from build123d import *

# Parameters (mm, degrees)
BOX001_W          = 40
BOX001_H          = 15
BOX001_DEPTH      = 5
CYLINDER003_R     = 3
CYLINDER003_DEPTH = 6
CYLINDER002_R     = 3
CYLINDER002_DEPTH = 6
CYLINDER001_R     = 1.7
CYLINDER001_DEPTH = 10
CYLINDER_R        = 1.7
CYLINDER_DEPTH    = 10
BOX_W             = 70
BOX_H             = 15
BOX_DEPTH         = 10
FILLET_R          = 2
FILLET001_R       = 2
FILLET002_R       = 7.45


with BuildPart() as cube001:
    # Box001 → Box001 (new body)
    with BuildSketch(Plane(origin=(15, 0, 5), x_dir=(1, 0, 0), z_dir=(0, 0, 1))):
        with Locations((20, 7.5)):
            Rectangle(BOX001_W, BOX001_H)
    extrude(amount=BOX001_DEPTH)


with BuildPart() as sphere001:
    # Sphere001 → Sphere001 (revolve)
    with BuildSketch(Plane(origin=(62.5, 7.5, -2), x_dir=(1, 0, 0), z_dir=(0, -1, 0))):
        with BuildLine():
            ThreePointArc((0, -5), (5, 0), (0, 5))
            Line((0, 5), (0, -5))
        make_face()
    revolve(axis=Axis((62.5, 7.5, -2), (0, 0, 1)))


with BuildPart() as sphere:
    # Sphere → Sphere (revolve)
    with BuildSketch(Plane(origin=(7.5, 7.5, -2), x_dir=(1, 0, 0), z_dir=(0, -1, 0))):
        with BuildLine():
            ThreePointArc((0, -5), (5, 0), (0, 5))
            Line((0, 5), (0, -5))
        make_face()
    revolve(axis=Axis((7.5, 7.5, -2), (0, 0, 1)))


with BuildPart() as cylinder003:
    # Cylinder003 → Cylinder003 (new body)
    with BuildSketch(Plane(origin=(62.5, 7.5, 0), x_dir=(1, 0, 0), z_dir=(0, 0, 1))):
        Circle(CYLINDER003_R)
    extrude(amount=CYLINDER003_DEPTH)


with BuildPart() as cylinder002:
    # Cylinder002 → Cylinder002 (new body)
    with BuildSketch(Plane(origin=(7.5, 7.5, 0), x_dir=(1, 0, 0), z_dir=(0, 0, 1))):
        Circle(CYLINDER002_R)
    extrude(amount=CYLINDER002_DEPTH)


with BuildPart() as cylinder001:
    # Cylinder001 → Cylinder001 (new body)
    with BuildSketch(Plane(origin=(62.5, 7.5, 0), x_dir=(1, 0, 0), z_dir=(0, 0, 1))):
        Circle(CYLINDER001_R)
    extrude(amount=CYLINDER001_DEPTH)


with BuildPart() as cylinder:
    # Cylinder → Cylinder (new body)
    with BuildSketch(Plane(origin=(7.5, 7.5, 0), x_dir=(1, 0, 0), z_dir=(0, 0, 1))):
        Circle(CYLINDER_R)
    extrude(amount=CYLINDER_DEPTH)


with BuildPart() as obj1:
    # Box → Box (new body)
    with BuildSketch(Plane.XY):
        with Locations((35, 7.5)):
            Rectangle(BOX_W, BOX_H)
    extrude(amount=BOX_DEPTH)

    # Fillet
    fillet_edges = [obj1.edges().sort_by_distance(p)[0] for p in [
        (0, 0, 5),
        (0, 15, 5),
        (70, 0, 5),
        (70, 15, 5),
    ]]
    fillet(fillet_edges, radius=FILLET_R)

    # Fillet001
    fillet001_edges = [obj1.edges().sort_by_distance(p)[0] for p in [
        (0, 7.5, 0),
        (0.585786, 0.585786, 0),
        (0.585786, 14.414214, 0),
        (35, 0, 0),
        (35, 15, 0),
        (69.414214, 0.585786, 0),
        (69.414214, 14.414214, 0),
        (70, 7.5, 0),
    ]]
    fillet(fillet001_edges, radius=FILLET001_R)

    # Cut: cut Cylinder
    add(cylinder.part, mode=Mode.SUBTRACT)

    # Cut001: cut Cylinder001
    add(cylinder001.part, mode=Mode.SUBTRACT)

    # Cut002: cut Cylinder002
    add(cylinder002.part, mode=Mode.SUBTRACT)

    # Cut003: cut Cylinder003
    add(cylinder003.part, mode=Mode.SUBTRACT)

    # Cut004: cut Sphere
    add(sphere.part, mode=Mode.SUBTRACT)

    # Cut005: cut Sphere001
    add(sphere001.part, mode=Mode.SUBTRACT)

    # Cut006: cut Cube001
    add(cube001.part, mode=Mode.SUBTRACT)

    # Fillet002
    fillet002_edges = [obj1.edges().sort_by_distance(p)[0] for p in [
        (55, 0, 7.5),
        (15, 0, 7.5),
        (55, 15, 7.5),
        (15, 15, 7.5),
    ]]
    fillet(fillet002_edges, radius=FILLET002_R)


solid = obj1.part
Could you check a few things on this model? Use its own coordinates, in mm. A direction names the side the tool comes from. Round coordinates to 2 decimals unless told otherwise and drop trailing zeros. Write each loop counter-clockwise with the first axis right and the second up, starting at its lowest first coordinate (ties: lowest second). Pieces come first, ordered by that corner, then holes. Notation, with made-up numbers: (77.25, 72) - (94.25, 72) arc R18 ccw to (94.25, 98) - close; hole circle Ø1 at (8, 88.5). An arc over 180 degrees is marked (long way). Put each result on its own line as item: value. Start each with the question number.
(1) I need wall thicknesses on probe 1 along X at (y, z) = (7.5, 8.2); probe 2 along Y at (x, z) = (62.5, 7.65); probe 3 along Y at (x, z) = (62.5, 3.65). Which ranges of each line are inside material? Lowest first, please.
(2) For faces 4 (the flat face through (70, 7, 6)), 5 (the cylindrical face through (57.24, 12.876, 7.535)), 6 (the flat face through (9, 6, 6)), 7 (the cylindrical face through (12.76, 2.124, 7.535)), 8 (the cylindrical face through (35.46, 14.43, 0.6)), which set-ups out of +Z, -Z, +X, -X, +Y, -Y let a thin tool reach every point of the face, with its end or its side?
(3) I want a section at A-A, the plane z = 9. Please give me the cut outline in (x, y).
(4) Will these pins go through, and if not, where does the flat tip stop? pin 1 (4.5 mm diameter, centred on x = 62.5, y = 7.5, fed in from -Z); pin 2 (4.5 mm diameter, centred on x = 36.5, y = 10.5, fed in from +Z).
(5) I want a section at D-D, the plane x = 6.5. Please give me the cut outline in (y, z).
(6) Thinking about a two-plate mould opening in Y: for faces 1 (the flat face through (35, 8, 0)), 2 (the cylindrical face through (12.76, 12.876, 7.535)), 3 (the cylindrical face through (10.27, 6.35, 3.97)), which applies, released by +Y, released by -Y, zero draft, split by the parting line, or undercut?
(7) I want a section at C-C, the plane y = 8.5. Give the number of separate pieces and of enclosed holes in the cut face, plus the area to 3 significant figures.
(8) I want a section at B-B, the plane z = 4.25. Please give me the cut outline in (x, y).
Here are the results:
1. probe 1: x = 0 to 5.8, 9.2 to 15, 55 to 60.8, 64.2 to 70
1. probe 2: y = 0 to 5.8, 9.2 to 15
1. probe 3: y = 0 to 4.5, 10.5 to 15
2. face 4: +Z, -Z, +X, +Y, -Y
2. face 5: +Z, +Y
2. face 6: -Z
2. face 7: +Z, -Y
2. face 8: -Z, +X, -X, +Y
3. outline: (0, 2) arc R2 ccw to (2, 0) - (7.55, 0) arc R7.45 ccw to (15, 7.45) - (15, 7.55) arc R7.45 ccw to (7.55, 15) - (2, 15) arc R2 ccw to (0, 13) - close; (55, 7.45) arc R7.45 ccw to (62.45, 0) - (68, 0) arc R2 ccw to (70, 2) - (70, 13) arc R2 ccw to (68, 15) - (62.45, 15) arc R7.45 ccw to (55, 7.55) - close; hole circle Ø3.4 at (7.5, 7.5); hole circle Ø3.4 at (62.5, 7.5)
4. pin 1: stops at z = 6
4. pin 2: stops at z = 5
5. outline: (0, 2) arc R2 ccw to (2, 0) - (3.03, 0) arc R4.9 cw to (4.67, 2) - (4.67, 6) - (6.13, 6) - (6.13, 10) - (0, 10) - close; (8.87, 6) - (10.33, 6) - (10.33, 2) arc R4.9 cw to (11.97, 0) - (13, 0) arc R2 ccw to (15, 2) - (15, 10) - (8.87, 10) - close
6. face 1: zero draft
6. face 2: released by +Y
6. face 3: undercut
7. separate pieces: 3
7. enclosed holes: 0
7. area: 400 mm^2
8. outline: (0, 2) arc R2 ccw to (2, 0) - (68, 0) arc R2 ccw to (70, 2) - (70, 13) arc R2 ccw to (68, 15) - (2, 15) arc R2 ccw to (0, 13) - close; hole circle Ø6 at (7.5, 7.5); hole circle Ø6 at (62.5, 7.5)
